Check sheet for the modelled part. Datum: model origin and axes. Units: mm. A direction names the side the tool comes from. Give positions to 0.01 mm unless a question says otherwise; leave off trailing zeros. Write each loop counter-clockwise with the first axis right and the second up, starting at its lowest first coordinate (ties: lowest second). Pieces come first, ordered by that corner, then holes. Notation, with made-up numbers: (34.25, -6) - (73.25, -6) arc R21 cw to (73.25, 21) - close; hole circle Ø8 at (71.5, 27). An arc over 180 degrees is marked (long way). Return JSON: item names as keys, results as strings. Group by question number.
```python
from build123d import *

# Parameters (mm, degrees)
SKETCH1_W            = 57.6
SKETCH1_H            = 12.7
BOSS_EXTRUDE1_DEPTH  = 9.525
BOSS_EXTRUDE2_DEPTH  = 9.525
MIRROR2_COPY_1_DEPTH = 9.525
FILLET1_R            = 1
CUT_EXTRUDE1_DEPTH   = 10.525
SKETCH3_W            = 1.62
SKETCH3_H            = 12.7
CUT_EXTRUDE2_DEPTH   = 2
LPATTERN1_COUNT      = 4
LPATTERN1_PITCH      = 3.5
LPATTERN1_COL_COUNT  = 4
LPATTERN1_COL_PITCH  = 3.5


with BuildPart() as part:
    # Sketch1 → Boss-Extrude1 (new body)
    with BuildSketch(Plane(origin=(0, 0, 0), x_dir=(1, 0, 0), z_dir=(0, 1, 0))):
        Rectangle(SKETCH1_W, SKETCH1_H)
    extrude(amount=BOSS_EXTRUDE1_DEPTH)

    # Sketch2 → Boss-Extrude2 (add)
    with BuildSketch(Plane(origin=(0, 9.525, 0), x_dir=(1, 0, 0), z_dir=(0, 1, 0))):
        Polygon((-28.8, 4.7625), (-38.8, 4.7625), (-40.189474334, 6.746875), (-42.189474334, 6.746875), (-43.578948667, 4.7625), (-43.578948667, 2.38125), (-28.8, 2.38125), align=None)
    boss_extrude2 = extrude(amount=-BOSS_EXTRUDE2_DEPTH)

    # Mirror1: Boss-Extrude2 across plane
    add(boss_extrude2.mirror(Plane(origin=(0, 0, 0), x_dir=(0, 0, 1), z_dir=(1, 0, 0))))

    # Mirror2: Boss-Extrude2 across plane
    add(boss_extrude2.mirror(Plane.XY))

    # Mirror2 copy 1 sketch → Mirror2 copy 1 (add)
    with BuildSketch(Plane(origin=(0, 9.525, 0), x_dir=(-1, 0, 0), z_dir=(0, 1, 0))):
        Polygon((-28.8, 4.7625), (-38.8, 4.7625), (-40.189474334, 6.746875), (-42.189474334, 6.746875), (-43.578948667, 4.7625), (-43.578948667, 2.38125), (-28.8, 2.38125), align=None)
    extrude(amount=-MIRROR2_COPY_1_DEPTH)

    # Fillet1
    fillet1_edges = [part.edges().sort_by_distance(p)[0] for p in [
        (-28.8, 4.7625, -4.7625),
        (-28.8, 4.7625, -2.38125),
        (28.8, 4.7625, -4.7625),
        (28.8, 4.7625, -2.38125),
        (-28.8, 4.7625, 4.7625),
        (-28.8, 4.7625, 2.38125),
        (28.8, 4.7625, 4.7625),
        (28.8, 4.7625, 2.38125),
    ]]
    fillet(fillet1_edges, radius=FILLET1_R)

    # Sketch4 → Cut-Extrude1 (cut, through all)
    with BuildSketch(Plane(origin=(0, 9.525, 0), x_dir=(1, 0, 0), z_dir=(0, 1, 0))):
        with BuildLine():
            Line((-19.05, 3.175), (19.05, 3.175))
            ThreePointArc((19.05, 3.175), (22.225, 0), (19.05, -3.175))
            Line((19.05, -3.175), (-19.05, -3.175))
            ThreePointArc((-19.05, -3.175), (-22.225, 0), (-19.05, 3.175))
        make_face()
    extrude(amount=-CUT_EXTRUDE1_DEPTH, mode=Mode.SUBTRACT)

    # Sketch3 → Cut-Extrude2 (cut)
    with BuildSketch(Plane(origin=(0, 9.525, 0), x_dir=(1, 0, 0), z_dir=(0, 1, 0))):
        Rectangle(SKETCH3_W, SKETCH3_H)
    cut_extrude2 = extrude(amount=-CUT_EXTRUDE2_DEPTH, mode=Mode.SUBTRACT)

    # LPattern1: Cut-Extrude2 ×4
    with Locations(*[(-i * LPATTERN1_PITCH, 0, 0) for i in range(1, LPATTERN1_COUNT)]):
        add(cut_extrude2, mode=Mode.SUBTRACT)

    # LPattern1 col: Cut-Extrude2 ×4
    with Locations(*[(i * LPATTERN1_COL_PITCH, 0, 0) for i in range(1, LPATTERN1_COL_COUNT)]):
        add(cut_extrude2, mode=Mode.SUBTRACT)


solid = part.part
```
Item 1: Access from +Z, -Z, +X, -X, +Y, -Y to the whole of each face (thin tool, end or side, straight path). Record for faces 4 (the face through (-28.8, 5, 0)), 5 (the face through (0, 5, -6.35)), 6 (the face through (6.19, 9, 5)), 7 (the face through (-2, 9.525, -5)), 8 (the face through (-34, 5, 4.762)).
Item 2: Depth check by flat-ended pin: pin 1 (4.5 mm diameter, centred on x = -32.5, y = 3.5, fed in from -Z); pin 2 (5 mm diameter, centred on x = -4.5, y = 3, fed in from -Z); pin 3 (0.8 mm diameter, centred on y = 6.5, z = 0.5, fed in from -X). Enter the tip coordinate at first touch or a pass-through.
Item 3: Material ranges on line 1 along Z through (x, y) = (-30.5, 1.75); line 2 along Z through (x, y) = (10, 2.75) (3 decimals); line 3 along X through (y, z) = (1.75, 6.25), recorded low to high. Write a range as from..to.
Item 4: Section check B-B on y = 8.5. Count the separate pieces of the cut face and the enclosed holes in it, plus the area to 3 significant figures.
Item 5: Mould release check, pull along Z, two halves, no side actions. Record for faces 1 (the face through (9.69, 9, 5)), 2 (the face through (28.8, 5, 0)), 3 (the face through (39.485, 4.829, 5.741)): +Z half, -Z half, draft (parallel to the pull), parting line (faces both ways), or undercut.
Item 6: Section check A-A on z = 0. Record the cut outline in (x, y) (3 decimals), plus the area to 3 significant figures.
Reply:
{
 "1": {"face 4": "-X, +Y, -Y", "face 5": "-Z, +Y, -Y", "face 6": "+Z, -Z, +Y", "face 7": "+Z, -Z, +X, -X, +Y", "face 8": "+Z, +Y, -Y"},
 "2": {"pin 1": "z = -4.76", "pin 2": "z = -6.35", "pin 3": "x = -28.8"},
 "3": {"line 1": "-4.76..-2.38, 2.38..4.76", "line 2": "-6.35..-3.175, 3.175..6.35", "line 3": "-42.54..-39.84, -28.8..28.8, 39.84..42.54"},
 "4": {"separate pieces": "14", "enclosed holes": "0", "area": "555 mm²"},
 "5": {"face 1": "draft", "face 2": "undercut", "face 3": "+Z half"},
 "6": {"outline": "(-28.8, 0) - (-22.225, 0) - (-22.225, 9.525) - (-28.8, 9.525) - close; (22.225, 0) - (28.8, 0) - (28.8, 9.525) - (22.225, 9.525) - close", "area": "125 mm²"}
}
